CAD build for the part. Positions are in the model's coordinates, mm. A direction names the side the tool comes from. Coordinates: 2 decimals unless noted, no trailing zeros. Write each loop counter-clockwise with the first axis right and the second up, starting at its lowest first coordinate (ties: lowest second). Pieces come first, ordered by that corner, then holes. Notation, with made-up numbers: (-30.5, 49) - (16.5, 49) arc R28 ccw to (16.5, 73) - close; hole circle Ø10 at (-8, 38.25). An arc over 180 degrees is marked (long way). One line per question, with ' | ' between items. Start each with the question number.
1. Band-saw the part on A-A, the plane z = 1.15. Write the cut outline in (x, y).
2. Flat gauge pins, fed straight in: P1, Ø1.8, axis at x = 20, y = 2, coming from the +Z side; P2, Ø1, axis at y = 3, z = 4.5, coming from the -X side. Where does each tip first touch, or does it go through?
3. Band-saw the part on C-C, the plane x = 39. Write the cut outline in (y, z), then the cut area to 3 significant figures.
4. Which spindle directions (+Z, -Z, +X, -X, +Y, -Y) get a long thin tool onto all of the face, cutting with end or side? Do faces 5 (the flat face through (27, 4.4, 3.7)), 6 (the flat face through (16, 0, 2)), 7 (the flat face through (18, 3, 2)). Say none if no direction does.
5. Probe line 1 (X direction, y = 2.5, z = 2.2); line 2 (X direction, y = 3.8, z = 4.55); line 3 (Z direction, x = 23.5, y = 4.95). List the from-to ranges inside material, lowest first.
6. Band-saw the part on D-D, the plane y = 5.3. Write the cut outline in (x, z), then the cut area to 3 significant figures.
7. Two-plate mould, pull along X, no slides. Class faces 1 (the flat face through (39, 3, 5.7)), 2 (the flat face through (9, 3, 0.2)), 3 (the flat face through (42, 3, 2)), 4 (the flat face through (33, 3, 0.2)): +X half, -X half, draft (parallel to the pull), parting line (faces both ways), or undercut.
Autodesk Fusion 360 part; units mm, degrees
sketch "Sketch1" plane through (0, 0, 0) normal (0, 0, 1) x (1, 0, 0)
  line L0 (0, 0) -> (6, 0)
  line L1 (6, 0) -> (6, 6)
  line L2 (6, 6) -> (0, 6)
  line L3 (0, 6) -> (0, 0)
  line L4 (12, 0) -> (18, 0)
  line L5 (18, 0) -> (18, 6)
  line L6 (18, 6) -> (12, 6)
  line L7 (12, 6) -> (12, 0)
  line L8 (24, 0) -> (30, 0)
  line L9 (30, 0) -> (30, 6)
  line L10 (30, 6) -> (24, 6)
  line L11 (24, 6) -> (24, 0)
  line L12 (36, 0) -> (42, 0)
  line L13 (42, 0) -> (42, 6)
  line L14 (42, 6) -> (36, 6)
  line L15 (36, 6) -> (36, 0)
  line L16 (0, 0) -> (42, 0)
  line L17 (42, 0) -> (42, 6)
  line L18 (42, 6) -> (0, 6)
  line L19 (0, 6) -> (0, 0)
  circle A0 centre (3, 3) radius 1.25
  circle A1 centre (15, 3) radius 1.25
  circle A2 centre (27, 3) radius 1.25
  circle A3 centre (39, 3) radius 1.25
  dimension "d1" = 6
  dimension "d2" = 6
  dimension "d5" = 6
  dimension "d6" = 6
  dimension "d7" = 6
  dimension "d8" = 6
  dimension "d9" = 6
  dimension "d10" = 6
  dimension "d11" = 6
  dimension "d12" = 6
  dimension "d13" = 6
  dimension "d18" = 2.5
  dimension "d19" = 2.5
  dimension "d20" = 2.5
  dimension "d21" = 2.5
extrude "Extrude2" add sketch "Sketch1" along normal blind 0.2 contours L0 L1 L2 L3 L16 L18 L19 | L1 L7 L16 L18 | L4 L5 L6 L7 L16 L18 | L5 L11 L16 L18 | L8 L9 L10 L11 L16 L18 | L9 L15 L16 L18 | L12 L13 L14 L15 L16 L17 L18 | A0 | A1 | A2 | A3
extrude "Extrude3" add sketch "Sketch1" along normal blind 3.7 contours L0 L1 L2 L3 L16 L18 L19 | L4 L5 L6 L7 L16 L18 | L8 L9 L10 L11 L16 L18 | L12 L13 L14 L15 L16 L17 L18 | A0 | A1 | A2 | A3
extrude "Extrude4" add sketch "Sketch1" along normal blind 5.7 contours A0 | A1 | A2 | A3
Filled in:
1) outline: (0, 0) - (6, 0) - (6, 6) - (0, 6) - close; (12, 0) - (18, 0) - (18, 6) - (12, 6) - close; (24, 0) - (30, 0) - (30, 6) - (24, 6) - close; (36, 0) - (42, 0) - (42, 6) - (36, 6) - close
2) P1: stops at z = 0.2 | P2: stops at x = 1.75
3) outline: (0, 0) - (6, 0) - (6, 3.7) - (4.25, 3.7) - (4.25, 5.7) - (1.75, 5.7) - (1.75, 3.7) - (0, 3.7) - close | area: 27.2 mm²
4) face 5: +Z | face 6: +Z, -Z, +X, -X, -Y | face 7: +Z, +Y, -Y
5) line 1: x = 0 to 6, 12 to 18, 24 to 30, 36 to 42 | line 2: x = 2.04 to 3.96, 14.04 to 15.96, 26.04 to 27.96, 38.04 to 39.96 | line 3: z = 0 to 0.2
6) outline: (0, 0) - (42, 0) - (42, 3.7) - (36, 3.7) - (36, 0.2) - (30, 0.2) - (30, 3.7) - (24, 3.7) - (24, 0.2) - (18, 0.2) - (18, 3.7) - (12, 3.7) - (12, 0.2) - (6, 0.2) - (6, 3.7) - (0, 3.7) - close | area: 92.4 mm²
7) face 1: draft | face 2: undercut | face 3: +X half | face 4: undercut
